Geometry check sheet. Reference: drawing and pictorial views, mm from the part's lowest x, y, z. A direction names the side the tool comes from. Round coordinates to 2 decimals unless told otherwise and drop trailing zeros. Order: outer loops, then holes, each group sorted by start corner. A loop starts at its lowest first (then second) coordinate and runs counter-clockwise, first axis right, second up.
Q1. Depth check by flat-ended pin: P1, Ø8, axis at x = 14.135, z = 14.135, coming from the +Y side; P2, Ø5, axis at y = 12, z = 6, coming from the +X side; P3, Ø1.5, axis at y = 9, z = 20, coming from the -X side; P4, Ø2, axis at y = 8, z = 24.5, coming from the +X side. Enter the tip coordinate at first touch or a pass-through.
Q2. Cross-section at B-B on x = 15. Record the cut outline in (y, z), then the cut area to 3 significant figures.
Q3. Mould release check, pull along Y, two halves, no side actions. Record for the marked faces 3, 4 and 5: +Y half, -Y half, draft (parallel to the pull), parting line (faces both ways), or undercut.
Q4. Set-up check for the marked faces 1 and 2: record each of +Z, -Z, +X, -X, +Y, -Y from which the full face is reachable in a straight line by a thin tool's end or side.
Q5. Cross-section at A-A on z = 17.5. Record the cut outline in (x, y).
Q6. Cross-section at D-D on x = 19.75. Record the cut outline in (y, z).
Q7. Scan lines: probe 1 along Y at (x, z) = (6.75, 3.25); probe 2 along Z at (x, y) = (5.25, 0.5); probe 3 along X at (y, z) = (6, 11.75). Record each from-to range of solid material in increasing order.
Q8. Cross-section at C-C on z = 22.5. Record the cut outline in (x, y).
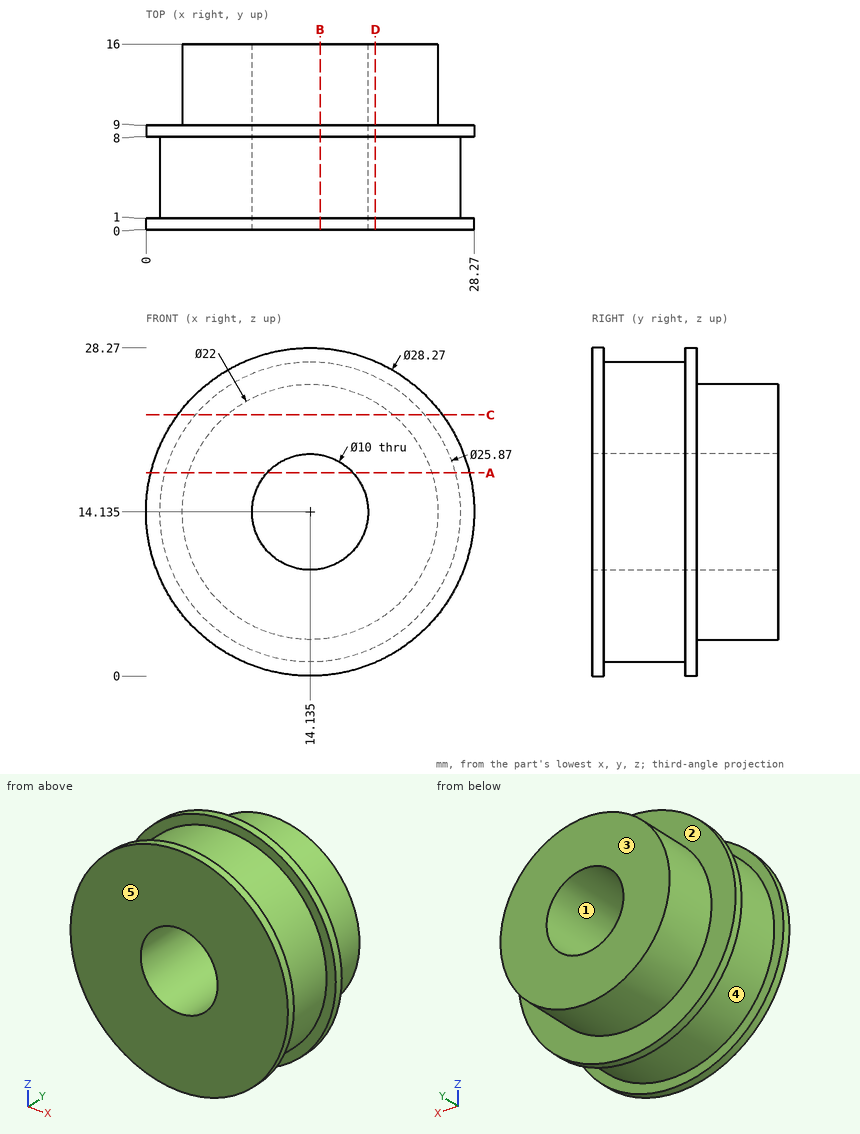
Results found:
1. P1: passes through
1. P2: stops at x = 23.58
1. P3: stops at x = 0.96
1. P4: stops at x = 24.72
2. outline: (0, 0.03) - (1, 0.03) - (1, 1.23) - (8, 1.23) - (8, 0.03) - (9, 0.03) - (9, 3.17) - (16, 3.17) - (16, 9.21) - (0, 9.21) - close; (0, 19.06) - (16, 19.06) - (16, 25.1) - (9, 25.1) - (9, 28.24) - (8, 28.24) - (8, 27.04) - (1, 27.04) - (1, 28.24) - (0, 28.24) - close
2. area: 233 mm2
3. face 3: +Y half
3. face 4: undercut
3. face 5: -Y half
4. face 1: +Y, -Y
4. face 2: +Y
5. outline: (0.41, 0) - (10.44, 0) - (10.44, 16) - (3.66, 16) - (3.66, 9) - (0.41, 9) - (0.41, 8) - (1.65, 8) - (1.65, 1) - (0.41, 1) - close; (17.83, 0) - (27.86, 0) - (27.86, 1) - (26.62, 1) - (26.62, 8) - (27.86, 8) - (27.86, 9) - (24.61, 9) - (24.61, 16) - (17.83, 16) - close
6. outline: (0, 1.16) - (1, 1.16) - (1, 2.48) - (8, 2.48) - (8, 1.16) - (9, 1.16) - (9, 4.68) - (16, 4.68) - (16, 23.59) - (9, 23.59) - (9, 27.11) - (8, 27.11) - (8, 25.79) - (1, 25.79) - (1, 27.11) - (0, 27.11) - close
7. probe 1: y = 0 to 1, 8 to 9
7. probe 2: z = 3.14 to 25.13
7. probe 3: x = 1.42 to 9.74, 18.53 to 26.85
8. outline: (2.74, 0) - (25.53, 0) - (25.53, 1) - (24, 1) - (24, 8) - (25.53, 8) - (25.53, 9) - (21.28, 9) - (21.28, 16) - (6.99, 16) - (6.99, 9) - (2.74, 9) - (2.74, 8) - (4.27, 8) - (4.27, 1) - (2.74, 1) - close
